Verification items for the finished model (mm, model axes). A direction names the side the tool comes from. Coordinates: 2 decimals unless noted, no trailing zeros. Loops run counter-clockwise (first coordinate to the right, second up) from the corner with the lowest first, then second, coordinate; pieces in that order, holes last. Notation, with made-up numbers: (-12, -14.5) - (36, -14.5) arc R15 cw to (36, -8.5) - close; hole circle Ø7 at (55, 66.5). An arc over 180 degrees is marked (long way). One line per item, written item: value. Start each with the question number.
(1) Thickness scan on probe 1 along Y at (x, z) = (-9, -32); probe 2 along Z at (x, y) = (-16, 57.75); probe 3 along Y at (x, z) = (-15.5, 32). Record the ranges inside material, lowest first. Write a range as [from, to].
(2) Section check C-C (y = 61.75). Record the boundary of the cut face in (x, z).
(3) Section check B-B (y = 56.75). Record the boundary of the cut face in (x, z), plus the area to 3 significant figures.
(4) Set-up check for faces 1 (the face through (-1, 58.428, -24)), 2 (the face through (-1, 55.428, 8)), 3 (the face through (0, 57, -21)), 4 (the face through (1, 59, 0)), 5 (the face through (0, 63.428, 12)): record each of +Z, -Z, +X, -X, +Y, -Y from which the full face is reachable in a straight line by a thin tool's end or side.
(5) Gauge pin test, flat ends, axial feed: P1, Ø3, axis at x = -10, y = 58, coming from the +Z side; P2, Ø12, axis at x = 28, z = -23, coming from the +Y side; P3, Ø4, axis at y = 57.5, z = 10, coming from the +X side. Record the tip position at first contact, or that the pin passes through.
(6) Section check A-A (x = 0). Record the boundary of the cut face in (y, z), plus the area to 3 significant figures.
```python
from build123d import *

# Parameters (mm, degrees)
CUT_EXTRUDE3_DEPTH           = 60
CUT_EXTRUDE5_DEPTH           = 2
CUT_EXTRUDE5_DEPTH_BACK      = 30
SKETCH19_W                   = 12
SKETCH19_H                   = 36.5
CUT_REVOLVE2_ANGLE           = 65
CUT_REVOLVE2_OTHER_WAY_ANGLE = 65
SKETCH21_W                   = 3.25
SKETCH21_H                   = 4
BOSS_EXTRUDE3_DEPTH          = 1.35
CIRPATTERN1_COUNT            = 5
CUT_EXTRUDE9_START           = -5
CUT_EXTRUDE9_DEPTH           = 5
INTERSECT1_DEPTH             = 55.427876097
INTERSECT1_START             = 55.427876097
INTERSECT1_2_OUTLINE_R       = 37.002145429
INTERSECT1_2_DEPTH           = 2


# Read off the part's stored shape, not the designer's step: Cut-Extrude9, Intersect1
with BuildPart() as part:
    # Sketch1 → Revolve1 (revolve)
    with BuildSketch(Plane.XY, mode=Mode.PRIVATE) as revolve1_sk:
        with BuildLine():
            Line((0, 63.427876097), (32, 63.427876097))
            ThreePointArc((32, 63.427876097), (37.656854249, 61.084730346), (40, 55.427876097))
            Line((40, 55.427876097), (40, 31.556288966))
            ThreePointArc((40, 31.556288966), (38.188122658, 24.409721904), (33.190210564, 18.989648567))
            Line((33.190210564, 18.989648567), (28.539859624, 15.958818353))
            ThreePointArc((28.539859624, 15.958818353), (25.207918228, 12.345436129), (24, 7.581058088))
            Line((24, 7.581058088), (24, 3.25))
            Line((24, 3.25), (24.35, 3))
            Line((24.35, 3), (24.35, 0))
            Line((24.35, 0), (22.5, 0))
            Line((22.5, 0), (22.5, 12.5))
            ThreePointArc((22.5, 12.5), (22.353553391, 12.853553391), (22, 13))
            Line((22, 13), (0, 13))
            Line((0, 13), (0, 63.427876097))
        make_face()
    revolve(revolve1_sk.sketch.rotate(Axis((0, 0, 0), (0, 1, 0)), 90), axis=Axis((0, 0, 0), (0, 1, 0)))

    # Sketch11 → Cut-Extrude3 (cut)
    with BuildSketch(Plane(origin=(0, 13, 0), x_dir=(-1, 0, 0), z_dir=(0, -1, 0))):
        with BuildLine():
            Line((-21, 0), (21, 0))
            ThreePointArc((21, 0), (0, 21), (-21, 0))
        make_face()
    extrude(amount=-CUT_EXTRUDE3_DEPTH, mode=Mode.SUBTRACT)

    # Sketch9 → Cut-Extrude5 (cut, two sides: drawn at the far end of the back side and taken through both)
    with BuildSketch(Plane(origin=(0, 55.427876097, 0), x_dir=(1, 0, 0), z_dir=(0, 1, 0)).offset(-CUT_EXTRUDE5_DEPTH_BACK)):
        with BuildLine():
            ThreePointArc((-37, -1.601545046), (-0.398454954, -39), (37, -2.398454954))
            ThreePointArc((37, -2.398454954), (0.398454954, 35), (-37, -1.601545046))
        make_face()
        with BuildLine():
            Line((-24, -1.763080838), (24, -1.763080838))
            ThreePointArc((24, -1.763080838), (0, 24), (-24, -1.763080838))
        make_face(mode=Mode.SUBTRACT)
    extrude(amount=CUT_EXTRUDE5_DEPTH + CUT_EXTRUDE5_DEPTH_BACK, mode=Mode.SUBTRACT)

    # Sketch19 → Cut-Revolve2 (revolve, cut)
    with BuildSketch(Plane(origin=(0, 0, 0), x_dir=(0, 0, -1), z_dir=(1, 0, 0))):
        with Locations((-41.064715832, 37.177876097)):
            Rectangle(SKETCH19_W, SKETCH19_H)
    revolve(axis=Axis((0, 0, 0), (0, 1, 0)), revolution_arc=CUT_REVOLVE2_ANGLE, mode=Mode.SUBTRACT)

    # Sketch19 → Cut-Revolve2 other way (revolve, cut)
    with BuildSketch(Plane(origin=(0, 0, 0), x_dir=(0, 0, -1), z_dir=(1, 0, 0))):
        with Locations((-41.064715832, 37.177876097)):
            Rectangle(SKETCH19_W, SKETCH19_H)
    revolve(axis=Axis((0, 0, 0), (0, -1, 0)), revolution_arc=CUT_REVOLVE2_OTHER_WAY_ANGLE, mode=Mode.SUBTRACT)

    # Sketch21 → Boss-Extrude3 (add)
    with BuildSketch(Plane(origin=(0, 0, 22.5), x_dir=(-1, 0, 0), z_dir=(0, 0, -1))):
        with Locations((0, 2)):
            Rectangle(SKETCH21_W, SKETCH21_H)
    boss_extrude3 = extrude(amount=BOSS_EXTRUDE3_DEPTH)

    # CirPattern1: Boss-Extrude3 ×5 about axis
    cirpattern1_axis = Axis((0, 0, 0), (0, 1, 0))
    for i in range(1, CIRPATTERN1_COUNT):
        add(boss_extrude3.rotate(cirpattern1_axis, i * 360 / CIRPATTERN1_COUNT))

    # Cut-Extrude9 outline → Cut-Extrude9 (cut)
    with BuildSketch(Plane(origin=(0, 63.427876097, 0), x_dir=(1, 0, 0), z_dir=(0, 1, 0)).offset(CUT_EXTRUDE9_START)):
        with BuildLine():
            ThreePointArc((40, 0), (0, 40), (-40, 0))
            Line((-40, 0), (-21, 0))
            ThreePointArc((-21, 0), (0, 21), (21, 0))
            Line((21, 0), (40, 0))
        make_face()
    extrude(amount=CUT_EXTRUDE9_DEPTH, mode=Mode.SUBTRACT)

    # Intersect1 outline → Intersect1 (cut)
    with BuildSketch(Plane(origin=(0, 0, 0), x_dir=(1, 0, 0), z_dir=(0, 1, 0))):
        with BuildLine():
            Line((31.779425009, -14.818989253), (36.252311481, -16.90473047))
            ThreePointArc((36.252311481, -16.90473047), (0, 40), (-36.252311481, -16.90473047))
            Line((-36.252311481, -16.90473047), (-31.779425009, -14.818989253))
            ThreePointArc((-31.779425009, -14.818989253), (0, -35.064715832), (31.779425009, -14.818989253))
        make_face()
        with BuildLine():
            ThreePointArc((-21, 0), (0, 21), (21, 0))
            Line((21, 0), (-21, 0))
        make_face(mode=Mode.SUBTRACT)
    extrude(amount=INTERSECT1_DEPTH, mode=Mode.SUBTRACT)

    # Intersect1 2 outline → Intersect1 2 (add)
    with BuildSketch(Plane(origin=(0, 0, 0), x_dir=(1, 0, 0), z_dir=(0, 1, 0)).offset(INTERSECT1_START)):
        with Locations((0, -2)):
            Circle(INTERSECT1_2_OUTLINE_R)
        with BuildLine():
            ThreePointArc((-24, -1.763080838), (0, 24), (24, -1.763080838))
            Line((24, -1.763080838), (-24, -1.763080838))
        make_face(mode=Mode.SUBTRACT)
    extrude(amount=INTERSECT1_2_DEPTH)


solid = part.part
```
Responses:
1. probe 1: y = [55.43, 58.43]
1. probe 2: z = [-36.28, -13.6], [0, 36.28]
1. probe 3: y = [55.43, 62.59]
2. outline: (-36.9, 0) - (36.9, 0) arc R36.9 ccw to start
3. outline: circle Ø79.78 at (0, 0); hole (-21, 0) arc R21 ccw to (21, 0) - close
3. area: 4,310 mm²
4. face 1: -Z, +X, -X, +Y
4. face 2: +Z, -Z, +X, -X, -Y
4. face 3: +Y, -Y
4. face 4: +Y
4. face 5: +Z, -Z, +X, -X, +Y
5. P1: stops at z = 38.84
5. P2: stops at y = 58.43
5. P3: stops at x = 39.06
6. outline: (55.43, -40) arc R8 ccw to (58.43, -39.42) - (58.43, -21) - (55.43, -21) - close; (55.43, 0) - (63.43, 0) - (63.43, 32) arc R8 ccw to (55.43, 40) - close
6. area: 363 mm²
